Work out the finished part from the listing and answer in its coordinate system (mm). A direction names the side the tool comes from. Coordinates: 2 decimals unless noted, no trailing zeros. Order: outer loops, then holes, each group sorted by start corner. A loop starts at its lowest first (then second) coordinate and runs counter-clockwise, first axis right, second up. Notation, with made-up numbers: (33.25, 20) -> (62.25, 20) arc R27 cw to (62.25, 52) -> close; hole circle Ø3 at (75, 29.25). An arc over 180 degrees is marked (long way). Answer as CSV lines item,"result". Start each with the question number.
Item 1: Section C-C (z = -72.5) is taken. Write down the section's boundary in (x, y) (3 decimals).
Item 2: Section B-B (z = -52.5) is taken. Write down the section's boundary in (x, y) (3 decimals).
Item 3: Each of these flat-tipped pins is pushed along its axis until it touches: pin 1 Ø1 at (x, z) = (138.5, -57.5) entering from +Y; pin 2 Ø5.5 at (x, z) = (120, -53) entering from +Y; pin 3 Ø1.3 at (x, z) = (63.5, -89.5) entering from +Y. Where does it stop, or does it pass through?
Item 4: Which of the six approach directions +Z, -Z, +X, -X, +Y, -Y give full straight-line access (tool end or side, diameter ignored) to faces 4 (the face through (147.263, 3, -60)), 5 (the face through (106, 0, -74))?
Item 5: Section A-A (x = 99) is taken. Write down the section's boundary in (y, z), then the cut area to 3 significant figures.
Item 6: Straight lines are drawn through the part: L1, parallel to Z at x = 66, y = 3.45; L2, parallel to X at y = 2.6, z = -68.5 (3 decimals); L3, parallel to X at y = 2.15, z = -59 (3 decimals). For each, find the intervals that lie inside material, in ascending order.
Item 7: For a pull along Z with two mould halves and no side action, classify faces 1 (the face through (105, 3, -46.736)), 2 (the face through (135, 2, -99.511)), 3 (the face through (62.865, 3, -74)) as pulls with the +Z half, pulls with the -Z half, needs draft (parallel to the pull), parting line crosses it, or undercut.
Item 8: Section D-D (y = 4.55) is taken. Count the separate pieces of the cut face and the enclosed holes in it, then the cut area to 3 significant figures.
```python
from build123d import *

# Parameters (mm, degrees)
BOSS_EXTRUDE1_DEPTH = 0.8
BOSS_EXTRUDE2_DEPTH = 5
SKETCH4_W           = 10
SKETCH4_H           = 3.2
CUT_EXTRUDE1_DEPTH  = 1.2
SKETCH6_W           = 6
SKETCH6_H           = 5
CUT_EXTRUDE2_DEPTH  = 1.2
SKETCH7_W           = 13
SKETCH7_H           = 3
CUT_EXTRUDE3_DEPTH  = 1.2
SKETCH8_R           = 2.7
SKETCH8_R_2         = 1.5
BOSS_EXTRUDE4_DEPTH = 5
SKETCH9_R           = 2.7
SKETCH9_R_2         = 1.5
BOSS_EXTRUDE5_DEPTH = 5
SKETCH10_R          = 2.7
SKETCH10_R_2        = 1.5
BOSS_EXTRUDE6_DEPTH = 5
SKETCH11_R          = 2.7
SKETCH11_R_2        = 1.5
BOSS_EXTRUDE7_DEPTH = 5
SKETCH13_R          = 2.3
CUT_EXTRUDE8_DEPTH  = 5
SKETCH15_W          = 41.2
SKETCH15_H          = 7.14
BOSS_EXTRUDE9_DEPTH = 1.2
SKETCH16_R          = 2.3
CUT_EXTRUDE9_DEPTH  = 40


with BuildPart() as part:
    # Sketch1 → Boss-Extrude1 (new body)
    with BuildSketch(Plane(origin=(0, 0, 0), x_dir=(1, 0, 0), z_dir=(0, 1, 0))):
        with BuildLine():
            Line((62.865, 49.276), (62.865, 98.171))
            ThreePointArc((62.865, 98.171), (63.608948776, 99.967051224), (65.405, 100.711))
            Line((65.405, 100.711), (145.923, 100.711))
            ThreePointArc((145.923, 100.711), (147.719051224, 99.967051224), (148.463, 98.171))
            Line((148.463, 98.171), (148.463, 49.276))
            ThreePointArc((148.463, 49.276), (147.719051224, 47.479948776), (145.923, 46.736))
            Line((145.923, 46.736), (65.405, 46.736))
            ThreePointArc((65.405, 46.736), (63.608948776, 47.479948776), (62.865, 49.276))
        make_face()
    extrude(amount=BOSS_EXTRUDE1_DEPTH)

    # Sketch3 → Boss-Extrude2 (add)
    with BuildSketch(Plane(origin=(0, 0.8, 0), x_dir=(1, 0, 0), z_dir=(0, 1, 0))):
        with BuildLine():
            Line((65.405, 46.736), (145.923, 46.736))
            ThreePointArc((145.923, 46.736), (147.719051224, 47.479948776), (148.463, 49.276))
            Line((148.463, 49.276), (148.463, 98.171))
            ThreePointArc((148.463, 98.171), (147.719051224, 99.967051224), (145.923, 100.711))
            Line((145.923, 100.711), (65.405, 100.711))
            ThreePointArc((65.405, 100.711), (63.608948776, 99.967051224), (62.865, 98.171))
            Line((62.865, 98.171), (62.865, 49.276))
            ThreePointArc((62.865, 49.276), (63.608948776, 47.479948776), (65.405, 46.736))
        make_face()
        with BuildLine():
            Line((64.065, 98.171), (64.065, 49.276))
            ThreePointArc((64.065, 49.276), (64.457476913, 48.328476913), (65.405, 47.936))
            Line((65.405, 47.936), (145.923, 47.936))
            ThreePointArc((145.923, 47.936), (146.870523087, 48.328476913), (147.263, 49.276))
            Line((147.263, 49.276), (147.263, 98.171))
            ThreePointArc((147.263, 98.171), (146.870523087, 99.118523087), (145.923, 99.511))
            Line((145.923, 99.511), (65.405, 99.511))
            ThreePointArc((65.405, 99.511), (64.457476913, 99.118523087), (64.065, 98.171))
        make_face(mode=Mode.SUBTRACT)
    extrude(amount=BOSS_EXTRUDE2_DEPTH)

    # Sketch4 → Cut-Extrude1 (cut)
    with BuildSketch(Plane.ZY.offset(-62.865)):
        with Locations((-90.011, 4.2)):
            Rectangle(SKETCH4_W, SKETCH4_H)
    extrude(amount=-CUT_EXTRUDE1_DEPTH, mode=Mode.SUBTRACT)

    # Sketch6 → Cut-Extrude2 (cut)
    with BuildSketch(Plane(origin=(0, 0, -100.711), x_dir=(-1, 0, 0), z_dir=(0, 0, -1))):
        with Locations((-122.963, 3.3)):
            Rectangle(SKETCH6_W, SKETCH6_H)
    extrude(amount=-CUT_EXTRUDE2_DEPTH, mode=Mode.SUBTRACT)

    # Sketch7 → Cut-Extrude3 (cut)
    with BuildSketch(Plane(origin=(0, 0, -100.711), x_dir=(-1, 0, 0), z_dir=(0, 0, -1))):
        with Locations((-136.063, 4.3)):
            Rectangle(SKETCH7_W, SKETCH7_H)
    extrude(amount=-CUT_EXTRUDE3_DEPTH, mode=Mode.SUBTRACT)

    # Sketch8 → Boss-Extrude4 (add)
    with BuildSketch(Plane(origin=(0, 0.8, 0), x_dir=(1, 0, 0), z_dir=(0, 1, 0))):
        with Locations((66.015, 97.486)):
            Circle(SKETCH8_R)
        with Locations(Location((66.015, 97.486, 0), (0, 0, 270))):
            Circle(SKETCH8_R_2, mode=Mode.SUBTRACT)
    extrude(amount=BOSS_EXTRUDE4_DEPTH)

    # Sketch9 → Boss-Extrude5 (add)
    with BuildSketch(Plane(origin=(0, 0.8, 0), x_dir=(1, 0, 0), z_dir=(0, 1, 0))):
        with Locations((145.5, 97.5)):
            Circle(SKETCH9_R)
        with Locations(Location((145.5, 97.5, 0), (0, 0, 270))):
            Circle(SKETCH9_R_2, mode=Mode.SUBTRACT)
    extrude(amount=BOSS_EXTRUDE5_DEPTH)

    # Sketch10 → Boss-Extrude6 (add)
    with BuildSketch(Plane(origin=(0, 0.8, 0), x_dir=(1, 0, 0), z_dir=(0, 1, 0))):
        with Locations((66, 68.5)):
            Circle(SKETCH10_R)
        with Locations(Location((66, 68.5, 0), (0, 0, 270))):
            Circle(SKETCH10_R_2, mode=Mode.SUBTRACT)
    extrude(amount=BOSS_EXTRUDE6_DEPTH)

    # Sketch11 → Boss-Extrude7 (add)
    with BuildSketch(Plane(origin=(0, 0.8, 0), x_dir=(1, 0, 0), z_dir=(0, 1, 0))):
        with Locations((145.5, 68.5)):
            Circle(SKETCH11_R)
        with Locations(Location((145.5, 68.5, 0), (0, 0, 270))):
            Circle(SKETCH11_R_2, mode=Mode.SUBTRACT)
    extrude(amount=BOSS_EXTRUDE7_DEPTH)

    # Sketch13 → Cut-Extrude8 (cut)
    with BuildSketch(Plane(origin=(148.463, 0, 0), x_dir=(0, 0, -1), z_dir=(1, 0, 0))):
        with Locations(Location((51.576, 3.1, 0), (0, 0, 180))):
            Circle(SKETCH13_R)
    extrude(amount=-CUT_EXTRUDE8_DEPTH, mode=Mode.SUBTRACT)

    # Sketch15 → Boss-Extrude9 (add)
    with BuildSketch(Plane(origin=(0, 0.8, 0), x_dir=(1, 0, 0), z_dir=(0, 1, 0))):
        with Locations((126.663, 51.506)):
            Rectangle(SKETCH15_W, SKETCH15_H)
    extrude(amount=BOSS_EXTRUDE9_DEPTH)

    # Sketch16 → Cut-Extrude9 (cut)
    with BuildSketch(Plane(origin=(147.263, 0, 0), x_dir=(0, 0, -1), z_dir=(1, 0, 0))):
        with Locations(Location((51.576, 3.1, 0), (0, 0, 180))):
            Circle(SKETCH16_R)
    extrude(amount=-CUT_EXTRUDE9_DEPTH, mode=Mode.SUBTRACT)


solid = part.part
```
Checked values:
1,outline,"(62.865, 0) -> (148.463, 0) -> (148.463, 5.8) -> (147.263, 5.8) -> (147.263, 0.8) -> (64.065, 0.8) -> (64.065, 5.8) -> (62.865, 5.8) -> close"
2,outline,"(62.865, 0) -> (148.463, 0) -> (148.463, 0.994) -> (107.263, 0.994) -> (107.263, 2) -> (106.063, 2) -> (106.063, 0.8) -> (64.065, 0.8) -> (64.065, 5.8) -> (62.865, 5.8) -> close; (147.263, 5.206) -> (148.463, 5.206) -> (148.463, 5.8) -> (147.263, 5.8) -> close"
3,pin 1,"stops at y = 0.8"
3,pin 2,"stops at y = 2"
3,pin 3,"stops at y = 2.6"
4,face 4,"+Y"
4,face 5,"+Z, -Z, +X, -X, -Y"
5,outline,"(0, -100.71) -> (5.8, -100.71) -> (5.8, -99.51) -> (0.8, -99.51) -> (0.8, -47.94) -> (5.8, -47.94) -> (5.8, -46.74) -> (0, -46.74) -> close"
5,area,"55.2 mm^2"
6,L1,"z = -100.71 to -98.99, -95.99 to -94.79, -71.2 to -70, -67 to -65.8, -47.94 to -46.74"
6,L2,"x = 62.865 to 64.5, 67.5 to 68.7, 142.8 to 144, 147 to 148.463"
6,L3,"x = 62.865 to 64.065, 147.263 to 148.463"
7,face 1,"pulls with the +Z half"
7,face 2,"undercut"
7,face 3,"needs draft"
8,separate pieces,"4"
8,enclosed holes,"4"
8,area,"336 mm^2"
